Answer from the drawing. Dimensions are ordinates in mm from the lowest x, y and z of the part. Round coordinates to 2 decimals unless told otherwise and drop trailing zeros. Write each loop counter-clockwise with the first axis right and the second up, starting at its lowest first coordinate (ties: lowest second). Pieces come first, ordered by that corner, then holes. Notation, with made-up numbers: (80.25, -14.75) - (94.25, -14.75) arc R20 cw to (94.25, -0.75) - close; hole circle Ø7 at (-21, 62). An arc over 180 degrees is marked (long way). Answer in a Markdown table with one row per item.
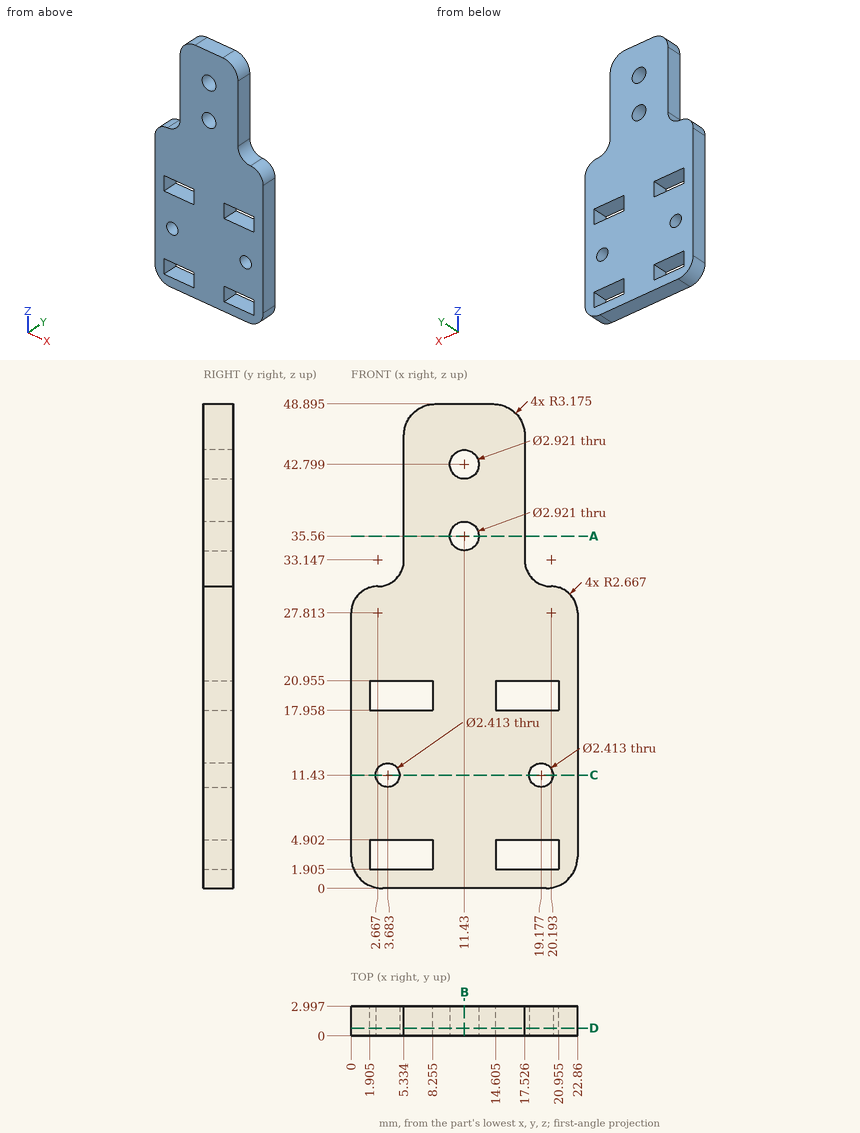
(1) Section A-A (z = 35.56) is taken. Give the vertices of the cut face in (x, y), and give its area (3 significant figures).
Checked values:
| item | result |
|---|---|
| outline | (5.33, 0) - (9.97, 0) - (9.97, 3) - (5.33, 3) - close; (12.89, 0) - (17.53, 0) - (17.53, 3) - (12.89, 3) - close |
| area | 27.8 mm2 |
(2) Find the intervals of material crossed by line 1 (X direction, y = 1.05, z = 11.43); line 2 (X direction, y = 0.7, z = 35.56); line 3 (Z direction, x = 17.75, y = 2.25) (1 decimal), in increasing order.
Checked values:
| item | result |
|---|---|
| line 1 | x = 0 to 2.48, 4.89 to 17.97, 20.38 to 22.86 |
| line 2 | x = 5.33 to 9.97, 12.89 to 17.53 |
| line 3 | z = 0 to 1.9, 4.9 to 18, 21 to 32.1 |
(3) Section D-D (y = 0.8) is taken. State how many separate pieces and enclosed holes the cut face has, and give its area (3 significant figures).
Checked values:
| item | result |
|---|---|
| separate pieces | 1 |
| enclosed holes | 8 |
| area | 814 mm2 |
(4) Section C-C (z = 11.43) is taken. Give the vertices of the cut face in (x, y).
Checked values:
| item | result |
|---|---|
| outline | (0, 0) - (2.48, 0) - (2.48, 3) - (0, 3) - close; (4.89, 0) - (17.97, 0) - (17.97, 3) - (4.89, 3) - close; (20.38, 0) - (22.86, 0) - (22.86, 3) - (20.38, 3) - close |
(5) Section B-B (x = 11.43) is taken. Give the vertices of the cut face in (y, z) (1 decimal), and give its area (3 significant figures).
Checked values:
| item | result |
|---|---|
| outline | (0, 0) - (3, 0) - (3, 34.1) - (0, 34.1) - close; (0, 37) - (3, 37) - (3, 41.3) - (0, 41.3) - close; (0, 44.3) - (3, 44.3) - (3, 48.9) - (0, 48.9) - close |
| area | 129 mm2 |
(6) Flat-ended cylindrical pins translate along their axes: pin 1 (0.9 mm diameter, centred on x = 16.5, y = 1, fed in from -Z); pin 2 (1.5 mm diameter, centred on x = 16.5, y = 2, fed in from +Z); pin 3 (1.5 mm diameter, centred on x = 3.5, y = 1, fed in from +Z). Find the tip coordinate at first contact, or state that the pin passes through.
Checked values:
| item | result |
|---|---|
| pin 1 | stops at z = 0 |
| pin 2 | stops at z = 48.57 |
| pin 3 | stops at z = 31 |
